Geometry: final body of the model. Coordinates: model frame, mm. Give positions to 0.01 mm unless a question says otherwise; leave off trailing zeros. Order: outer loops, then holes, each group sorted by start corner. A loop starts at its lowest first (then second) coordinate and runs counter-clockwise, first axis right, second up. Notation, with made-up numbers: (63, 68.5) -> (85, 68.5) arc R13 ccw to (85, 81.5) -> close; hole circle Ø6 at (-22.75, 16). An arc over 180 degrees is marked (long way). One line per question, with ' | ' between items.
Autodesk Inventor part; units mm, degrees
ref_plane "YZ Plane" through (0, 0, 0) normal (1, 0, 0) x (0, 1, 0)
ref_plane "XZ Plane" through (0, 0, 0) normal (0, 1, 0) x (-1, 0, 0)
ref_plane "XY Plane" through (0, 0, 0) normal (0, 0, 1) x (1, 0, 0)
sketch "草圖1" plane through (0, 0, 0) normal (0, 1, 0) x (-1, 0, 0)
  line L0 (3, 2.25) -> (-3, 2.25)
  line L1 (-3, 2.25) -> (-3, -2.25)
  line L2 (-3, -2.25) -> (3, -2.25)
  line L3 (3, -2.25) -> (3, 2.25)
  line L4 (3, 2.25) -> (-3, -2.25) construction
  line L5 (-3, 2.25) -> (3, -2.25) construction
  point P0 (0, 0)
  dimension "d0" = 6
  dimension "d1" = 4.5
extrude "擠出1" add sketch "草圖1" along normal blind 1.8
sketch "草圖2" plane through (-3, 0, 2.25) normal (0, 0, 1) x (1, 0, 0)
  line L0 (6, 0) -> (0, 0)
  line L1 (0, 0) -> (0.5, 0)
  line L2 (0.5, 0) -> (1.3, 0)
  line L3 (1.3, 0) -> (1.3, 0.5)
  line L4 (1.3, 0.5) -> (0.5, 0.5)
  line L5 (0.5, 0.5) -> (0.5, 0)
  point P0 (3, 0)
  point P1 (1.3, 0)
  dimension "d4" = 0.5
  dimension "d5" = 0.8
  dimension "d6" = 0.5
extrude "擠出2" add sketch "草圖2" along normal blind 2.2
pattern_linear "矩形陣列1" count 4 spacing 1.5 along (1, 0, 0) of "擠出2"
mirror "鏡射1" about plane through (0, 0, 0) normal (0, 0, 1) of "擠出2", "矩形陣列1"
ref_plane "工作平面1" through (-3, 1.8, 0) normal (0, 0, 1) x (1, 0, 0)
properties part number "鏡射"
1) Section A-A on z = 2.75. Return loops of the section in (x, y), plus the area to 3 significant figures.
Check result:
outline: (-2.5, 0) -> (-1.7, 0) -> (-1.7, 0.5) -> (-2.5, 0.5) -> close; (-1, 0) -> (-0.2, 0) -> (-0.2, 0.5) -> (-1, 0.5) -> close; (0.5, 0) -> (1.3, 0) -> (1.3, 0.5) -> (0.5, 0.5) -> close; (2, 0) -> (2.8, 0) -> (2.8, 0.5) -> (2, 0.5) -> close | area: 1.60 mm^2
2) Section B-B on x = -2.35. Return loops of the section in (y, z).
Check result:
outline: (0, -4.45) -> (0.5, -4.45) -> (0.5, -2.25) -> (1.8, -2.25) -> (1.8, 2.25) -> (0.5, 2.25) -> (0.5, 4.45) -> (0, 4.45) -> close
3) Section D-D on x = 0.3. Return loops of the section in (y, z), plus the area to 3 significant figures.
Check result:
outline: (0, -2.25) -> (1.8, -2.25) -> (1.8, 2.25) -> (0, 2.25) -> close | area: 8.10 mm^2
4) Pull-direction query (X, two-part tool) for faces 1 (the flat face through (0, 1.8, 0)), 2 (the flat face through (0, 1, -2.25)), 3 (the flat face through (-3, 1, 0)); classes: +X half, -X half, draft (parallel to the pull), parting line (faces both ways), or undercut.
Check result:
face 1: draft | face 2: undercut | face 3: -X half
5) Section C-C on y = 1.45. Return loops of the section in (x, z).
Check result:
outline: (-3, -2.25) -> (3, -2.25) -> (3, 2.25) -> (-3, 2.25) -> close
6) Contact query for flat-ended pins moving along their axis: pin 1 Ø0.6 at (y, z) = (0.5, -3) entering from -X; pin 2 Ø0.6 at (x, z) = (-0.5, 3) entering from +Y; pin 3 Ø0.5 at (x, y) = (0, 1) entering from -Z. Output: stop coordinate, or through.
Check result:
pin 1: stops at x = -2.5 | pin 2: stops at y = 0.5 | pin 3: stops at z = -2.25
7) Material intervals for probe 1 along X at (y, z) = (0.35, 2.5); probe 2 along Y at (x, z) = (0.8, 3.75); probe 3 along Z at (x, y) = (-2.05, 0.9), sorted ascending. Write a range as from..to.
Check result:
probe 1: x = -2.5..-1.7, -1..-0.2, 0.5..1.3, 2..2.8 | probe 2: y = 0..0.5 | probe 3: z = -2.25..2.25
